For this review, take the finished solid that the model builds, in its own axes (mm). A direction names the side the tool comes from. Give positions to 0.01 mm unless a question says otherwise; leave off trailing zeros. Order: outer loops, then holes, each group sorted by start corner. A loop starts at its lowest first (then second) coordinate and runs counter-clockwise, first axis right, second up. Notation, with made-up numbers: (75.25, 60.25) -> (133.25, 60.25) arc R16 ccw to (133.25, 72.25) -> close; hole circle Ø8 at (38, -33). An arc over 180 degrees is marked (long way). One line per item, written item: value. Start each with the question number.
Autodesk Inventor part; units mm, degrees
ref_plane "YZ Plane" through (0, 0, 0) normal (1, 0, 0) x (0, 1, 0)
ref_plane "XZ Plane" through (0, 0, 0) normal (0, 1, 0) x (-1, 0, 0)
ref_plane "XY Plane" through (0, 0, 0) normal (0, 0, 1) x (1, 0, 0)
sketch "Sketch1" plane through (0, 0, 0) normal (0, 0, 1) x (1, 0, 0)
  line L0 (-41.5, 50) -> (41.5, 50) construction
  line L1 (41.5, 50) -> (41.5, -50) construction
  line L2 (41.5, -50) -> (-41.5, -50) construction
  line L3 (-41.5, -50) -> (-41.5, 50) construction
  line L4 (0, 52.1292) -> (0, -48.3366) construction
  line L5 (-75.7124, 0) -> (96.9256, 0) construction
  circle A0 centre (-38.5, 47) radius 2.25
  line L6 (-31.25, 7) -> (0, 7)
  line L7 (0, 7) -> (0, -7)
  line L8 (0, -7) -> (-31.25, -7)
  line L9 (-31.25, -7) -> (-31.25, 7)
  circle A1 centre (-19, 0) radius 2.25
  line L10 (38.5, 47) -> (-38.5, 47) construction
  line L11 (-38.5, 47) -> (-38.5, -47) construction
  line L12 (-38.5, -47) -> (38.5, -47) construction
  line L13 (38.5, -47) -> (38.5, 47) construction
  circle A2 centre (38.5, 47) radius 2.25
  circle A3 centre (38.5, -47) radius 2.25
  circle A4 centre (-38.5, -47) radius 2.25
  line L14 (-31.25, -7) -> (-24.25, -7)
  line L15 (-24.25, -7) -> (-24.25, -37.6997)
  line L16 (-24.25, -37.6997) -> (-31.25, -37.6997)
  line L17 (-31.25, -37.6997) -> (-31.25, -7)
  line L18 (-44, -47.5503) -> (-39.0503, -52.5)
  line L19 (-39.0503, -52.5) -> (-24.25, -37.6997)
  line L20 (-24.25, -37.6997) -> (-29.1997, -32.75)
  line L21 (-29.1997, -32.75) -> (-44, -47.5503)
  line L22 (-26.7249, -35.2249) -> (-41.5251, -50.0251) construction
  line L23 (-41.5, -50) -> (-10.8193, -19.3193) construction
  line L24 (-41.5, -50) -> (1.8891, -50) construction
  line L25 (-35.5, -44) -> (-44, -44)
  line L26 (-44, -44) -> (-44, -52.5)
  line L27 (-44, -52.5) -> (-35.5, -52.5)
  line L28 (-35.5, -52.5) -> (-35.5, -44)
  circle A5 centre (-38.5, 0) radius 2.25
  line L29 (-31.25, 7) -> (-41.5, 7)
  line L30 (-41.5, 7) -> (-41.5, -7)
  line L31 (-41.5, -7) -> (-31.25, -7)
  line L32 (-31.25, -7) -> (-31.25, 7)
  point P0 (0, 0)
  point P1 (41.5, 0)
  point P2 (0, 50)
  dimension "d0" = 83
  dimension "d3" = 4.5
  dimension "d5" = 3
  dimension "d9" = 14
  dimension "d10" = 4.5
  dimension "d11" = 19
  dimension "d14" = 100
  dimension "d16" = 3
  dimension "d17" = 4.5
  dimension "d18" = 4.5
  dimension "d19" = 4.5
  dimension "d20" = 7
  dimension "d21" = 7
  dimension "d22" = 45
  dimension "d23" = 3
  dimension "d24" = 5.5
  dimension "d25" = 5.5
  dimension "d26" = 3
  dimension "d27" = 3
  dimension "d28" = 4.5
extrude "Extrusion1" add sketch "Sketch1" along normal blind 1.5 contours L6 L7 L8 L9 | L9 L31 L30 L29 | L8 L15 L20 L21 L17 | L21 L20 L16 L17 | L17 L16 L19 L28 L25 L21 | L25 L28 L19 L18 L21 | L21 L26 L25 | L28 L27 L19 | L18 L27 L26
mirror "Mirror1" about plane through (0, 0, 0) normal (1, 0, 0) of "Extrusion1"
mirror "Mirror2" about plane through (0, 0, 0) normal (0, 1, 0) of "Extrusion1", "Mirror1"
properties part number "MotorSideHolder"
Q1. Take a section at D-D (x = 32.5). State the section outline as (y, z) points, and give its area (3 significant figures).
Q2. For faces 5 (the flat face through (-35.79, -39.34, 0.74)), 6 (the flat face through (-29.95, -43.4, 0.74)), 7 (the flat face through (35.91, -39.46, 0.74)), 8 (the flat face through (29.95, 43.4, 0.74)), list the 3-axis set-ups (+Z, -Z, +X, -X, +Y, -Y) from which the entire face can be reached by the end or side of a thin tool; tool diameter is ignored.
Q3. For pin 1 Ø0.8 at (y, z) = (3.5, 1) entering from +X, flat-tipped, find the tip position at first contact; note if it passes through.
Q4. Take a section at A-A (y = -12.5). State the section outline as (x, z) points.
Q5. Mouldability with a two-part tool opening along X and no side actions: class faces 1 (the flat face through (0, -4, 1.5)), 2 (the flat face through (-29.8, 43.25, 0.74)), 3 (the cylindrical face through (38.79, 49.23, 0.74)), 4 (the flat face through (-35.91, 39.46, 0.74)) as pulls with the +X half, pulls with the -X half, needs draft (parallel to the pull), parting line crosses it, or undercut.
Q6. For line 1 along X through (y, z) = (-2, 1.2); line 2 along Y through (x, z) = (38.5, 1.2); line 3 along Y through (x, z) = (-32.5, 0.35), list the stretches that pass through material, from the lowest coordinate up.
Q7. Take a section at B-B (y = 0). State the section outline as (x, z) points.
Q8. Take a section at C-C (x = -19). State the section outline as (y, z) points, and give its area (4 significant figures).
Answers below:
1. outline: (-45.95, 0) -> (-36.05, 0) -> (-36.05, 1.5) -> (-45.95, 1.5) -> close; (-7, 0) -> (7, 0) -> (7, 1.5) -> (-7, 1.5) -> close; (36.05, 0) -> (45.95, 0) -> (45.95, 1.5) -> (36.05, 1.5) -> close
1. area: 50.7 mm²
2. face 5: +Z, -Z, -X
2. face 6: +Z, -Z, -Y
2. face 7: +Z, -Z, +X
2. face 8: +Z, -Z, +Y
3. pin 1: stops at x = 41.5
4. outline: (-31.25, 0) -> (-24.25, 0) -> (-24.25, 1.5) -> (-31.25, 1.5) -> close; (24.25, 0) -> (31.25, 0) -> (31.25, 1.5) -> (24.25, 1.5) -> close
5. face 1: needs draft
5. face 2: undercut
5. face 3: undercut
5. face 4: pulls with the -X half
6. line 1: x = -41.5 to -39.53, -37.47 to -20.03, -17.97 to 17.97, 20.03 to 37.47, 39.53 to 41.5
6. line 2: y = -52.5 to -49.25, -44.75 to -42.05, -7 to -2.25, 2.25 to 7, 42.05 to 44.75, 49.25 to 52.5
6. line 3: y = -45.95 to -36.05, -7 to 7, 36.05 to 45.95
7. outline: (-41.5, 0) -> (-40.75, 0) -> (-40.75, 1.5) -> (-41.5, 1.5) -> close; (-36.25, 0) -> (-21.25, 0) -> (-21.25, 1.5) -> (-36.25, 1.5) -> close; (-16.75, 0) -> (16.75, 0) -> (16.75, 1.5) -> (-16.75, 1.5) -> close; (21.25, 0) -> (36.25, 0) -> (36.25, 1.5) -> (21.25, 1.5) -> close; (40.75, 0) -> (41.5, 0) -> (41.5, 1.5) -> (40.75, 1.5) -> close
8. outline: (-7, 0) -> (-2.25, 0) -> (-2.25, 1.5) -> (-7, 1.5) -> close; (2.25, 0) -> (7, 0) -> (7, 1.5) -> (2.25, 1.5) -> close
8. area: 14.25 mm²
